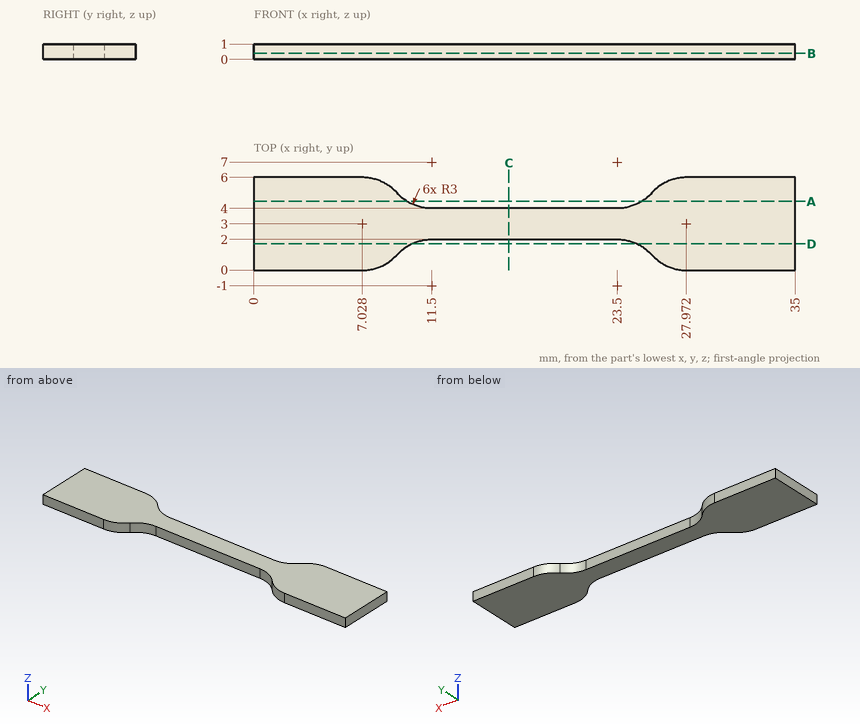
Here's the drawing with two shaded views (mm, measured from the low corner). I have some questions. Coordinates: 2 decimals unless noted, no trailing zeros. Write each loop counter-clockwise with the first axis right and the second up, starting at its lowest first coordinate (ties: lowest second). Pieces come first, ordered by that corner, then holes.
Item 1: I want a section at B-B on z = 0.4. Write out the boundary of the cut face in (x, y).
Item 2: I want a section at D-D on y = 1.7. Write out the boundary of the cut face in (x, z).
Item 3: I want a section at A-A on y = 4.45. Write out the boundary of the cut face in (x, z).
Item 4: I want a section at C-C on x = 16.5. Write out the boundary of the cut face in (y, z), and give its area (3 significant figures).
Item 5: If I drill on line 1 (X direction, y = 1, z = 0.85); line 2 (Y direction, x = 13, z = 0.35); line 3 (X direction, y = 0.4, z = 0.7) (1 decimal), over which ranges is the centre line in solid material (lowest first)?
Findings below:
1. outline: (0, 0) - (7.03, 0) arc R3 ccw to (9.26, 1) arc R3 cw to (11.5, 2) - (23.5, 2) arc R3 cw to (25.74, 1) arc R3 ccw to (27.97, 0) - (35, 0) - (35, 6) - (27.97, 6) arc R3 ccw to (25.74, 5) arc R3 cw to (23.5, 4) - (11.5, 4) arc R3 cw to (9.26, 5) arc R3 ccw to (7.03, 6) - (0, 6) - close
2. outline: (0, 0) - (10.19, 0) - (10.19, 1) - (0, 1) - close; (24.81, 0) - (35, 0) - (35, 1) - (24.81, 1) - close
3. outline: (0, 0) - (9.92, 0) - (9.92, 1) - (0, 1) - close; (25.08, 0) - (35, 0) - (35, 1) - (25.08, 1) - close
4. outline: (2, 0) - (4, 0) - (4, 1) - (2, 1) - close
4. area: 2.00 mm2
5. line 1: x = 0 to 9.26, 25.74 to 35
5. line 2: y = 2 to 4
5. line 3: x = 0 to 8.5, 26.5 to 35
